Design review of the part built by this model. Coordinates are the model's own, in mm. Face numbers are marked on the shaded views. A direction names the side the tool comes from. Coordinates: 2 decimals unless noted, no trailing zeros. One line per question, with ' | ' between items.
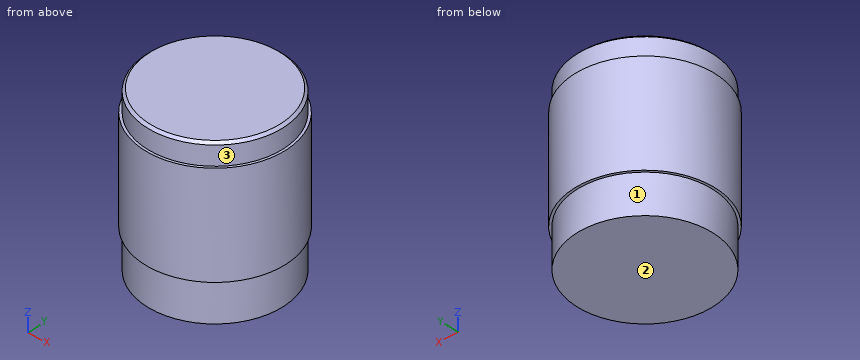
from build123d import *

# Parameters (mm, degrees)
BOSS_EXTRUDE1_START = 3.7
SKETCH2_R           = 6.95
BOSS_EXTRUDE1_DEPTH = 16.7
BOSS_EXTRUDE2_START = -9
SKETCH2_4_R         = 7.2
SKETCH2_4_R_2       = 6.95
BOSS_EXTRUDE2_DEPTH = 10.5
CHAMFER1_SIZE       = 0.25


with BuildPart() as part:
    # Sketch2 → Boss-Extrude1 (new body)
    with BuildSketch(Plane(origin=(0, -9.35e-07, 21.39999965), x_dir=(1, 0, 0), z_dir=(0, -4.4e-08, 1)).offset(BOSS_EXTRUDE1_START)):
        with Locations((6.560058174, 8.001830475)):
            Circle(SKETCH2_R)
        with BuildLine():
            Line((5.060057781, 10.246824644), (5.060058566, 5.75683578))
            ThreePointArc((5.060058566, 5.75683578), (9.260058174, 8.001830947), (5.060057781, 10.246824644))
        make_face(mode=Mode.SUBTRACT)
        with BuildLine():
            ThreePointArc((5.060058566, 5.75683578), (9.260058174, 8.001830947), (5.060057781, 10.246824644))
            Line((5.060057781, 10.246824644), (5.060058566, 5.75683578))
        make_face()
    extrude(amount=-BOSS_EXTRUDE1_DEPTH)

    # Sketch2_4 → Boss-Extrude2 (add)
    with BuildSketch(Plane(origin=(0, -9.35e-07, 21.39999965), x_dir=(1, 0, 0), z_dir=(0, -4.4e-08, 1)).offset(BOSS_EXTRUDE2_START)):
        with Locations((6.560058174, 8.001830475)):
            Circle(SKETCH2_4_R)
        with Locations((6.560058174, 8.001830475)):
            Circle(SKETCH2_4_R_2, mode=Mode.SUBTRACT)
    extrude(amount=BOSS_EXTRUDE2_DEPTH)

    # Chamfer1
    chamfer1_edges = [part.edges().sort_by_distance(p)[0] for p in [
        (-0.389941826, 8.001829378, 25.1),
    ]]
    chamfer(chamfer1_edges, length=CHAMFER1_SIZE)


solid = part.part
Q1. To check wall thickness, follow line 1 along Y through (x, z) = (6, 16.5); line 2 along Z through (x, y) = (13.25, 7); line 3 along Y through (x, z) = (6.25, 11.5). State the ranges of each line that lie inside material, in increasing order.
Returned:
line 1: y = 0.82 to 15.18 | line 2: z = 8.4 to 25.04 | line 3: y = 1.06 to 14.94
Q2. For pin 1 (1 mm diameter, centred on x = 9, z = 20, fed in from -Y); pin 2 (3 mm diameter, centred on x = 3.5, z = 17.5, fed in from +Y); pin 3 (2 mm diameter, centred on x = 5, z = 14.5, fed in from -Y), all flat-tipped, find the tip position at first contact; note any pin that passes through.
Returned:
pin 1: stops at y = 1.07 | pin 2: stops at y = 15.03 | pin 3: stops at y = 0.82
Q3. Tool access review of the marked faces 1, 2 and 3: name each direction out of +Z, -Z, +X, -X, +Y, -Y from which nothing blocks a thin tool from reaching the whole face with its end or side.
Returned:
face 1: -Z | face 2: -Z, +X, -X, +Y, -Y | face 3: +Z
